Read the model definition and answer for the solid it produces. Units are mm, in the model's axes. A direction names the side the tool comes from. Coordinates: 2 decimals unless noted, no trailing zeros. Write each loop counter-clockwise with the first axis right and the second up, starting at its lowest first coordinate (ties: lowest second). Pieces come first, ordered by that corner, then holes. Notation, with made-up numbers: M 64,64.5 L 113,64.5 A15 cw 113,81.5 Z; hole C -9,70 d8. An arc over 180 degrees is marked long. Write item = value, one per line.
from build123d import *

# Parameters (mm, degrees)
F0_R      = 603.25
F0_R_2    = 34.925
F1_DEPTH  = 50.8
F2_W      = 654.05
F2_H      = 654.05
F2_W_2    = 577.85
F2_H_2    = 577.85
F3_DEPTH  = 3.175
F4_W      = 654.05
F4_H      = 654.05
F4_W_2    = 647.7
F4_H_2    = 647.7
F5_DEPTH  = 34.925
F7_DEPTH  = 762
F9_DEPTH  = 762
F11_DEPTH = 762
F13_DEPTH = 762
F14_W     = 3.175
F14_H     = 3.175
F15_DEPTH = 34.925
F16_W     = 577.85
F16_H     = 577.85
F17_DEPTH = 3.175


with BuildPart() as f1:
    # F0 (on Top) → F1 (new body)
    with BuildSketch(Plane.XY):
        Circle(F0_R)
        Circle(F0_R_2, mode=Mode.SUBTRACT)
    extrude(amount=F1_DEPTH)

    # F2 (on face) → F3 (join)
    with BuildSketch(Plane(origin=(0, 0, 0), x_dir=(1, 0, 0), z_dir=(0, 0, -1))):
        Rectangle(F2_W, F2_H)
        Rectangle(F2_W_2, F2_H_2, mode=Mode.SUBTRACT)
    extrude(amount=F3_DEPTH)

    # F4 (on face) → F5 (join)
    with BuildSketch(Plane(origin=(0, 0, -3.175), x_dir=(1, 0, 0), z_dir=(0, 0, -1))):
        Rectangle(F4_W, F4_H)
        Rectangle(F4_W_2, F4_H_2, mode=Mode.SUBTRACT)
    extrude(amount=F5_DEPTH)

    # F6 (on face) → F7 (join)
    with BuildSketch(Plane(origin=(0, 0, -3.175), x_dir=(1, 0, 0), z_dir=(0, 0, -1))):
        Polygon((-285.75, 323.85), (-323.85, 323.85), (-323.85, 285.75), (-320.675, 285.75), (-320.675, 320.675), (-285.75, 320.675), align=None)
    extrude(amount=F7_DEPTH)

    # F8 (on face) → F9 (join)
    with BuildSketch(Plane(origin=(0, 0, -3.175), x_dir=(1, 0, 0), z_dir=(0, 0, -1))):
        Polygon((323.85, 285.75), (323.85, 323.85), (285.75, 323.85), (285.75, 320.675), (320.675, 320.675), (320.675, 285.75), align=None)
    extrude(amount=F9_DEPTH)

    # F10 (on face) → F11 (join)
    with BuildSketch(Plane(origin=(0, 0, -3.175), x_dir=(1, 0, 0), z_dir=(0, 0, -1))):
        Polygon((285.75, -323.85), (323.85, -323.85), (323.85, -285.75), (320.675, -285.75), (320.675, -320.675), (285.75, -320.675), align=None)
    extrude(amount=F11_DEPTH)

    # F12 (on face) → F13 (join)
    with BuildSketch(Plane(origin=(0, 0, -3.175), x_dir=(1, 0, 0), z_dir=(0, 0, -1))):
        Polygon((-323.85, -285.75), (-323.85, -323.85), (-285.75, -323.85), (-285.75, -320.675), (-320.675, -320.675), (-320.675, -285.75), align=None)
    extrude(amount=F13_DEPTH)

    # F14 (on face) → F15 (join)
    with BuildSketch(Plane(origin=(0, 0, -765.175), x_dir=(1, 0, 0), z_dir=(0, 0, -1))):
        with Locations((-325.4375, -325.4375)):
            Rectangle(F14_W, F14_H)
        Polygon((323.85, -323.85), (-323.85, -323.85), (-323.85, -327.025), (327.025, -327.025), (327.025, 323.85), (323.85, 323.85), align=None)
        Polygon((-327.025, -323.85), (-323.85, -323.85), (-323.85, 323.85), (323.85, 323.85), (323.85, 327.025), (-327.025, 327.025), align=None)
        with Locations((325.4375, 325.4375)):
            Rectangle(F14_W, F14_H)
    extrude(amount=-F15_DEPTH)

    # F16 (on face) → F17 (join)
    with BuildSketch(Plane(origin=(0, 0, -765.175), x_dir=(1, 0, 0), z_dir=(0, 0, -1))):
        Polygon((-327.025, -288.925), (-327.025, -327.025), (288.925, -327.025), (327.025, -327.025), (327.025, -288.925), (327.025, 327.025), (288.925, 327.025), (-288.925, 327.025), (-327.025, 327.025), align=None)
        Rectangle(F16_W, F16_H, mode=Mode.SUBTRACT)
    extrude(amount=F17_DEPTH)


solid = f1.part
Item 1: Flat-ended cylindrical pins translate along their axes: pin 1 (12 mm diameter, centred on x = 116.5, y = 470.5, fed in from -Z); pin 2 (17.5 mm diameter, centred on x = -132.5, z = -25, fed in from +Y) (3 decimals); pin 3 (3 mm diameter, centred on x = 315, z = -575.5, fed in from -Y); pin 4 (6 mm diameter, centred on x = -31, y = 0, fed in from -Z). Find the tip coordinate at first contact, or state that the pin passes through.
Worked answers:
pin_1 = 0
pin_2 = 327.025
pin_3 = -323.85
pin_4 = through
Item 2: Find section B-B (x = 0). State how many separate pieces and enclosed holes the cut face has, and give its area (3 significant figures).
Worked answers:
separate_pieces = 4
enclosed_holes = 0
area = 58,700 mm²
Item 3: Find section D-D (y = 206). Determine the outline of the cut face in (x, z) (3 decimals), and give its area (3 significant figures).
Worked answers:
outline = M -566.987,0 L -327.025,0 L -327.025,-38.1 L -323.85,-38.1 L -323.85,-3.175 L -288.925,-3.175 L -288.925,0 L 288.925,0 L 288.925,-3.175 L 323.85,-3.175 L 323.85,-38.1 L 327.025,-38.1 L 327.025,0 L 566.987,0 L 566.987,50.8 L -566.987,50.8 Z; M -327.025,-768.35 L -288.925,-768.35 L -288.925,-765.175 L -323.85,-765.175 L -323.85,-730.25 L -327.025,-730.25 Z; M 288.925,-768.35 L 327.025,-768.35 L 327.025,-730.25 L 323.85,-730.25 L 323.85,-765.175 L 288.925,-765.175 Z
area = 58,500 mm²
Item 4: Consider line 1 along X through (y, z) = (279, -35) (3 decimals); line 2 along Y through (x, z) = (0, 34) (3 decimals). Determine where each line is inside the solid, lowest interval first. Write a range as from..to.
Worked answers:
line_1 = -327.025..-323.85, 323.85..327.025
line_2 = -603.25..-34.925, 34.925..603.25
Item 5: Find section A-A (z = -198). Determine the outline of the cut face in (x, y) (3 decimals), and give its area (3 significant figures).
Worked answers:
outline = M -323.85,-323.85 L -285.75,-323.85 L -285.75,-320.675 L -320.675,-320.675 L -320.675,-285.75 L -323.85,-285.75 Z; M -323.85,285.75 L -320.675,285.75 L -320.675,320.675 L -285.75,320.675 L -285.75,323.85 L -323.85,323.85 Z; M 285.75,-323.85 L 323.85,-323.85 L 323.85,-285.75 L 320.675,-285.75 L 320.675,-320.675 L 285.75,-320.675 Z; M 285.75,320.675 L 320.675,320.675 L 320.675,285.75 L 323.85,285.75 L 323.85,323.85 L 285.75,323.85 Z
area = 927 mm²
Item 6: Which of the six approach directions +Z, -Z, +X, -X, +Y, -Y give full straight-line access (tool end or side, diameter ignored) to faces 1 (the face through (305, -323.85, -379)), 2 (the face through (-323.85, 305, -379)), 3 (the face through (-4, -323.85, -20)), 4 (the face through (5, -327.025, -749))?
Worked answers:
face_1 = +X, -X, -Y
face_2 = -X, +Y, -Y
face_3 = none
face_4 = -Z, +X, -X, -Y
Item 7: For a pull along Z with two mould halves and no side action, classify faces 5 (the face through (-5, 327.025, -19)), 6 (the face through (323.85, -305, -379)) as released by +Z, released by -Z, zero draft, split by the parting line, or undercut.
Worked answers:
face_5 = zero draft
face_6 = undercut
